Check sheet for the modelled part. Datum: model origin and axes. Units: mm. Face numbers are marked on the shaded views. A direction names the side the tool comes from. Round coordinates to 2 decimals unless told otherwise and drop trailing zeros. Loops run counter-clockwise (first coordinate to the right, second up) from the corner with the lowest first, then second, coordinate; pieces in that order, holes last. Notation, with made-up numbers: (52.5, 78) -> (66.5, 78) arc R20 cw to (66.5, 85) -> close; hole circle Ø2 at (-15.5, 1). An arc over 180 degrees is marked (long way). One line per question, with ' | ' between items.
```python
from build123d import *

# Parameters (mm, degrees)
SKETCH_W        = 65
SKETCH_H        = 45
PAD_DEPTH       = 24
SKETCH001_W     = 52.5
SKETCH001_H     = 29
POCKET_DEPTH    = 20
SKETCH002_R     = 1.7
SKETCH002_W     = 36.5
SKETCH002_H     = 29
POCKET001_DEPTH = 24.001
POCKET002_DEPTH = 3


with BuildPart() as part:
    # Sketch → Pad (new body)
    with BuildSketch(Plane.XY):
        with Locations((32.5, 22.5)):
            Rectangle(SKETCH_W, SKETCH_H)
    extrude(amount=PAD_DEPTH)

    # Sketch001 (on Face6 of Pad) → Pocket (cut)
    with BuildSketch(Plane.XY.offset(24)):
        with Locations((29.25, 22.5)):
            Rectangle(SKETCH001_W, SKETCH001_H)
    extrude(amount=-POCKET_DEPTH, mode=Mode.SUBTRACT)

    # Sketch002 (on Face5 of Pocket) → Pocket001 (cut, through all)
    with BuildSketch(Plane.XY.offset(24)):
        with Locations((3, 42)):
            Circle(SKETCH002_R)
        with Locations((62, 42)):
            Circle(SKETCH002_R)
        with Locations((62, 3)):
            Circle(SKETCH002_R)
        with Locations((3, 3)):
            Circle(SKETCH002_R)
        with Locations((29.25, 22.5)):
            Rectangle(SKETCH002_W, SKETCH002_H)
    extrude(amount=-POCKET001_DEPTH, mode=Mode.SUBTRACT)

    # Sketch003 (on Face2 of Pocket001) → Pocket002 (cut)
    with BuildSketch(Plane(origin=(0, 0, 0), x_dir=(0, -1, 0), z_dir=(-1, 0, 0))):
        with BuildLine():
            ThreePointArc((-27.5, 12), (-31.5, 8), (-27.5, 4))
            Line((-27.5, 4), (-17.5, 4))
            ThreePointArc((-17.5, 4), (-13.5, 8), (-17.5, 12))
            Line((-27.5, 12), (-17.5, 12))
        make_face()
    extrude(amount=-POCKET002_DEPTH, mode=Mode.SUBTRACT)


solid = part.part
```
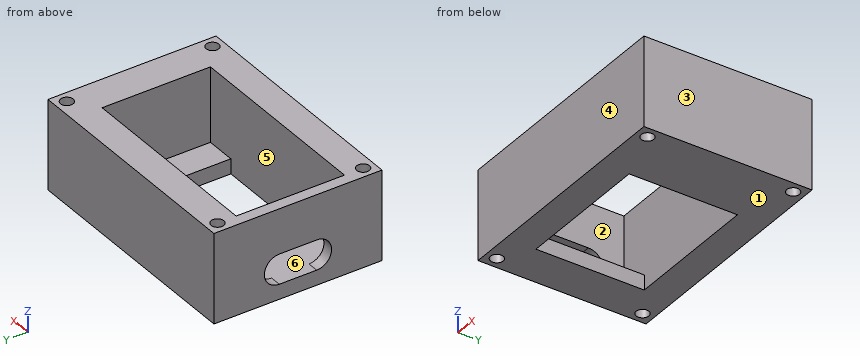
(1) Sectioned sample at B-B, the plane y = 42. Record the cut outline in (x, z), and give its area (3 significant figures).
Answer:
outline: (0, 0) -> (1.3, 0) -> (1.3, 24) -> (0, 24) -> close; (4.7, 0) -> (60.3, 0) -> (60.3, 24) -> (4.7, 24) -> close; (63.7, 0) -> (65, 0) -> (65, 24) -> (63.7, 24) -> close | area: 1,400 mm2
(2) Sectioned sample at D-D, the plane z = 8. Record the cut outline in (x, y).
Answer:
outline: (0, 0) -> (65, 0) -> (65, 45) -> (0, 45) -> (0, 31.5) -> (3, 31.5) -> (3, 37) -> (55.5, 37) -> (55.5, 8) -> (3, 8) -> (3, 13.5) -> (0, 13.5) -> close; hole circle Ø3.4 at (3, 3); hole circle Ø3.4 at (3, 42); hole circle Ø3.4 at (62, 3); hole circle Ø3.4 at (62, 42)
(3) Sectioned sample at C-C, the plane z = 17. Record the cut outline in (x, y).
Answer:
outline: (0, 0) -> (65, 0) -> (65, 45) -> (0, 45) -> close; hole circle Ø3.4 at (3, 3); hole circle Ø3.4 at (3, 42); hole (3, 8) -> (55.5, 8) -> (55.5, 37) -> (3, 37) -> close; hole circle Ø3.4 at (62, 3); hole circle Ø3.4 at (62, 42)
(4) Go/stop test with a flat-tipped pin: pin 1 (4 mm diameter, centred on x = 52, y = 23.5, fed in from +Z). Record where the tip stops, or that it passes through.
Answer:
pin 1: stops at z = 4
(5) Scan lines: probe 1 along Y at (x, z) = (62, 15.75); probe 2 along Y at (x, z) = (27.5, 16.75); probe 3 along X at (y, z) = (11, 10). Record each from-to range of solid material in increasing order.
Answer:
probe 1: y = 0 to 1.3, 4.7 to 40.3, 43.7 to 45 | probe 2: y = 0 to 8, 37 to 45 | probe 3: x = 0 to 3, 55.5 to 65
(6) Set-up check for the marked faces 1 and 2: record each of +Z, -Z, +X, -X, +Y, -Y from which the full face is reachable in a straight line by a thin tool's end or side.
Answer:
face 1: -Z, +X, -X, +Y, -Y | face 2: +Z
(7) Mould release check, pull along Y, two halves, no side actions. Record for the marked faces 3, 4, 5 and 6: +Y half, -Y half, draft (parallel to the pull), parting line (faces both ways), or undercut.
Answer:
face 3: draft | face 4: -Y half | face 5: undercut | face 6: undercut
(8) Sectioned sample at A-A, the plane x = 30. Record the cut outline in (y, z).
Answer:
outline: (0, 0) -> (8, 0) -> (8, 24) -> (0, 24) -> close; (37, 0) -> (45, 0) -> (45, 24) -> (37, 24) -> close
